from build123d import *

# Parameters (mm, degrees)
BOX_W             = 10.7
BOX_H             = 6
BOX_DEPTH         = 0.4
CYLINDER_R        = 5
CYLINDER_DEPTH    = 0.4
CYLINDER001_R     = 4.15
CYLINDER001_DEPTH = 12
FILLET_R          = 0.75
CYLINDER002_R     = 3.3
CYLINDER002_DEPTH = 10
FILLET001_R       = 0.2
BOX001_W          = 1.5
BOX001_H          = 0.4
BOX001_DEPTH      = 10.1
BOX002_W          = 0.4
BOX002_H          = 6
BOX002_DEPTH      = 3.8
BOX003_W          = 0.4
BOX003_H          = 6
BOX003_DEPTH      = 3.8


with BuildPart() as part:
    # Box → Box (join)
    with BuildSketch(Plane(origin=(-5.35, -3, 0), x_dir=(1, 0, 0), z_dir=(0, 0, 1))):
        with Locations((5.35, 3)):
            Rectangle(BOX_W, BOX_H)
    extrude(amount=BOX_DEPTH)

    # Cylinder → Cylinder (join)
    with BuildSketch(Plane.XY):
        Circle(CYLINDER_R)
    extrude(amount=CYLINDER_DEPTH)

    # Cylinder001 → Cylinder001 (join)
    with BuildSketch(Plane.XY):
        Circle(CYLINDER001_R)
    extrude(amount=CYLINDER001_DEPTH)

    # Fillet
    fillet_edges = [part.edges().sort_by_distance(p)[0] for p in [
        (-4.15, 0, 12),
    ]]
    fillet(fillet_edges, radius=FILLET_R)

    # Cylinder002 → Cylinder002 (cut)
    with BuildSketch(Plane.XY.offset(2)):
        Circle(CYLINDER002_R)
    extrude(amount=CYLINDER002_DEPTH, mode=Mode.SUBTRACT)

    # Fillet001
    fillet001_edges = [part.edges().sort_by_distance(p)[0] for p in [
        (-3.3, 0, 12),
    ]]
    fillet(fillet001_edges, radius=FILLET001_R)

    # Box001 → Box001 (join)
    with BuildSketch(Plane(origin=(-0.75, 1.4, -10.1), x_dir=(1, 0, 0), z_dir=(0, 0, 1))):
        with Locations((0.75, 0.2)):
            Rectangle(BOX001_W, BOX001_H)
    extrude(amount=BOX001_DEPTH)

    # Box002 → Box002 (join)
    with BuildSketch(Plane(origin=(4.95, -3, -3.4), x_dir=(1, 0, 0), z_dir=(0, 0, 1))):
        with Locations((0.2, 3)):
            Rectangle(BOX002_W, BOX002_H)
    extrude(amount=BOX002_DEPTH)

    # Box003 → Box003 (join)
    with BuildSketch(Plane(origin=(-5.35, -3, -3.4), x_dir=(1, 0, 0), z_dir=(0, 0, 1))):
        with Locations((0.2, 3)):
            Rectangle(BOX003_W, BOX003_H)
    extrude(amount=BOX003_DEPTH)


solid = part.part
Can you work these out from the model? Positions are in its coordinate system, mm. A direction names the side the tool comes from. Coordinates: 2 decimals unless noted, no trailing zeros. Loops run counter-clockwise (first coordinate to the right, second up) from the corner with the lowest first, then second, coordinate; pieces in that order, holes last. Notation, with made-up numbers: (28, 76) - (73, 76) arc R29 cw to (73, 110) - close; hole circle Ø11 at (48, 70.5). An arc over 180 degrees is marked (long way). Answer as a JSON object with one key per item and string values. Group by question number.
Item 1: On a 3-axis mill with a long thin cutter (end or side, diameter ignored), from which of +Z, -Z, +X, -X, +Y, -Y can I reach the whole of each face in a straight line? I mean faces 1 (the face through (-5.1, 3, -1.1)), 2 (the face through (-4.95, 0, -2)), 3 (the face through (-5.1, -3, -1.1)). Say none if no direction works.
Item 2: If we section it at C-C (z = -4.25): List the corners of the cut face in (x, y) for me.
Item 3: If we section it at B-B (z = 6.75): List the corners of the cut face in (x, y) for me, plus the area to 3 significant figures.
Item 4: For pin 1 (0.8 mm diameter, centred on x = 0, z = -3.5, fed in from -Y); pin 2 (2 mm diameter, centred on y = 1.5, z = 6, fed in from +X); pin 3 (1.5 mm diameter, centred on x = -2.5, y = 0, fed in from +Z), each with a flat end and sliding along its axis, tell me the tip position at first contact or that it passes through.
Item 5: If we mould it in two halves opening along X, with no side actions, what happens to faces 4 (the face through (0, 0, 2)), 5 (the face through (0.1, 5, 0.2)), 6 (the face through (4.95, 0, -2)), 7 (the face through (-2, -4, 0.4))? For each: released by +X, released by -X, zero draft, split by the parting line, or undercut.
Item 6: If we section it at A-A (z = -0.25): List the corners of the cut face in (x, y) for me, plus the area to 3 significant figures.
Item 7: If I drill on L1, parallel to Y at x = 0, z = 8.25; L2, parallel to Z at x = -4.5, y = -0.5, over which ranges is the centre line in solid material (lowest first)? Write a range as from..to.
Returned:
{
 "1": {"face 1": "+Z, -Z, -X, +Y", "face 2": "-Z, +Y, -Y", "face 3": "+Z, -Z, -X, -Y"},
 "2": {"outline": "(-0.75, 1.4) - (0.75, 1.4) - (0.75, 1.8) - (-0.75, 1.8) - close"},
 "3": {"outline": "circle Ø8.3 at (0, 0); hole circle Ø6.6 at (0, 0)", "area": "19.9 mm²"},
 "4": {"pin 1": "stops at y = 1.4", "pin 2": "stops at x = 4.12", "pin 3": "stops at z = 2"},
 "5": {"face 4": "undercut", "face 5": "split by the parting line", "face 6": "undercut", "face 7": "zero draft"},
 "6": {"outline": "(-5.35, -3) - (-4.95, -3) - (-4.95, 3) - (-5.35, 3) - close; (-0.75, 1.4) - (0.75, 1.4) - (0.75, 1.8) - (-0.75, 1.8) - close; (4.95, -3) - (5.35, -3) - (5.35, 3) - (4.95, 3) - close", "area": "5.40 mm²"},
 "7": {"L1": "y = -4.15..-3.3, 3.3..4.15", "L2": "z = 0..0.4"}
}
